Source: three-view drawing plus pictorial views. Frame: mm from the lowest corner of the part. Round coordinates to 2 decimals unless told otherwise and drop trailing zeros. Write each loop counter-clockwise with the first axis right and the second up, starting at its lowest first coordinate (ties: lowest second). Pieces come first, ordered by that corner, then holes. Notation, with made-up numbers: M 21,-16.5 L 63,-16.5 A8 ccw 63,-12.5 Z; hole C 51,-38.75 d7. An arc over 180 degrees is marked long. Answer in a Markdown table with one row per item.
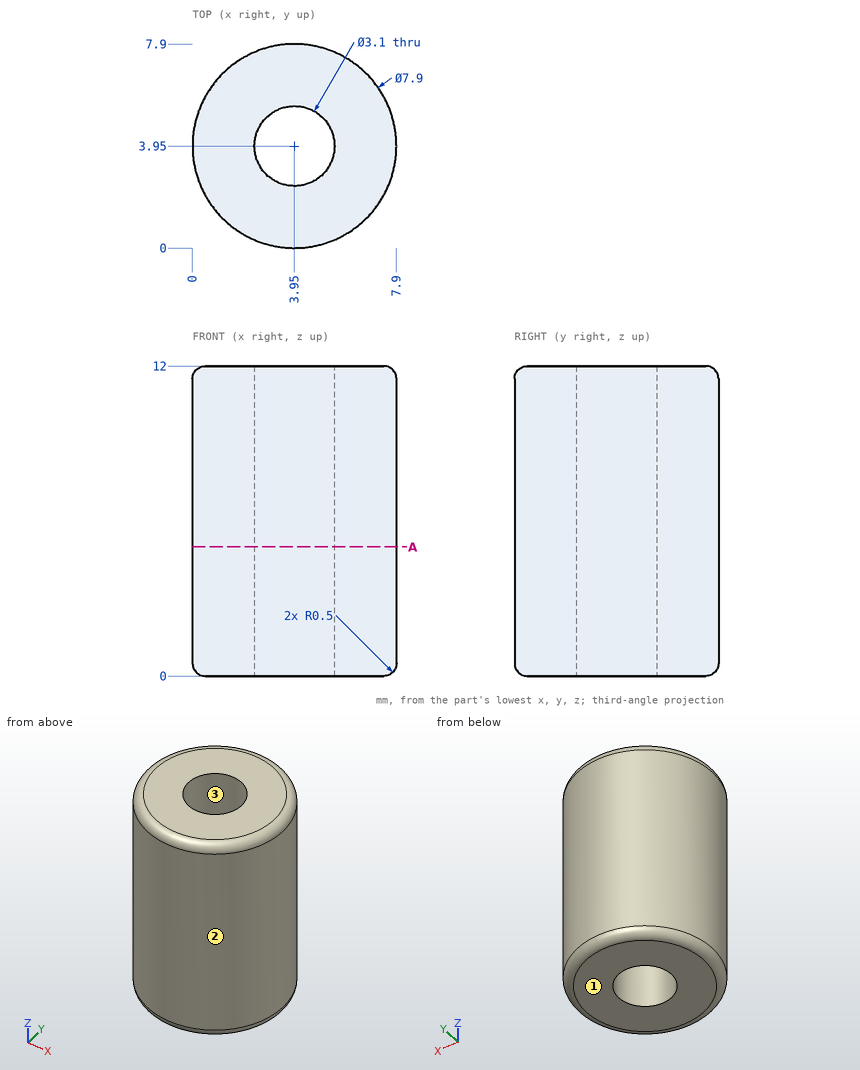
Q1. Section A-A (z = 5). Return loops of the section in (x, y), and give its area (3 significant figures).
Solutions:
| item | result |
|---|---|
| outline | C 3.95,3.95 d7.9; hole C 3.95,3.95 d3.1 |
| area | 41.5 mm2 |
Q2. Pull-direction query (X, two-part tool) for the marked faces 1, 2 and 3; classes: pulls with the +X half, pulls with the -X half, needs draft (parallel to the pull), parting line crosses it, or undercut.
Solutions:
| item | result |
|---|---|
| face 1 | needs draft |
| face 2 | parting line crosses it |
| face 3 | undercut |
Q3. Contact query for a flat-ended pin moving along its axis: pin 1 Ø3 at (x, z) = (6, 10.5) entering from +Y. Output: stop coordinate, or through.
Solutions:
| item | result |
|---|---|
| pin 1 | stops at y = 7.86 |
Q4. Material intervals for probe 1 along Y at (x, z) = (3.95, 3.5); probe 2 along Y at (x, z) = (5, 5.25); probe 3 along X at (y, z) = (4.25, 3.75), sorted ascending.
Solutions:
| item | result |
|---|---|
| probe 1 | y = 0 to 2.4, 5.5 to 7.9 |
| probe 2 | y = 0.14 to 2.81, 5.09 to 7.76 |
| probe 3 | x = 0.01 to 2.43, 5.47 to 7.89 |
